Autodesk Inventor part; units mm, degrees
ref_plane "YZ Plane" through (0, 0, 0) normal (1, 0, 0) x (0, 1, 0)
ref_plane "XZ Plane" through (0, 0, 0) normal (0, 1, 0) x (-1, 0, 0)
ref_plane "XY Plane" through (0, 0, 0) normal (0, 0, 1) x (1, 0, 0)
sketch "Sketch1" plane through (0, 0, 0) normal (0, 1, 0) x (-1, 0, 0)
  circle A0 centre (0, 0) radius 36
  circle A1 centre (0, 0) radius 29
  line L0 (0, 0) -> (32.313, 0)
  circle A2 centre (32.313, 0) radius 1.25
  circle A3 centre (16.1565, 27.9839) radius 1.25
  circle A4 centre (-16.1565, 27.9839) radius 1.25
  circle A5 centre (-32.313, 0) radius 1.25
  circle A6 centre (-16.1565, -27.9839) radius 1.25
  circle A7 centre (16.1565, -27.9839) radius 1.25
  dimension "d0" = 72
  dimension "d1" = 58
  dimension "d2" = 32.313
  dimension "d3" = 2.5
  dimension "d6" = 360
extrude "Extrusion1" add sketch "Sketch1" along normal blind 15
sketch "Sketch2" plane through (0, 15, 0) normal (0, 1, 0) x (1, 0, 0)
  circle A0 centre (0, 0) radius 29
  circle A1 centre (0, 0) radius 31.063
  circle A2 centre (-16.1565, 27.9839) radius 1.25
  circle A3 centre (0, 0) radius 36
  point P0 (-15.5315, 26.9013)
extrude "Extrusion2" cut sketch "Sketch2" against normal blind 10 contours A3
sketch "Sketch3" plane through (0, 15, 0) normal (0, 1, 0) x (1, 0, 0)
  circle A0 centre (0, 0) radius 31.063
  circle A1 centre (0, 0) radius 8.5
  dimension "d12" = 17
extrude "Extrusion3" add sketch "Sketch3" along normal blind 3
sketch "Sketch4" plane through (0, 18, 0) normal (0, 1, 0) x (1, 0, 0)
  circle A0 centre (-32.313, 0) radius 1.25
  circle A1 centre (-32.313, 0) radius 3
  circle A2 centre (0, 0) radius 8.5
  circle A3 centre (-16.1565, -27.9839) radius 3
  circle A4 centre (16.1565, -27.9839) radius 3
  circle A5 centre (32.313, 0) radius 3
  circle A6 centre (16.1565, 27.9839) radius 3
  circle A7 centre (-16.1565, 27.9839) radius 3
  dimension "d15" = 6
  dimension "d18" = 360
extrude "Extrusion4" cut sketch "Sketch4" against normal up to surface (13 mm away) contours A0 | A1 | A3 | A4 | A5 | A6 | A7
properties part number "Stage_1_Lid"
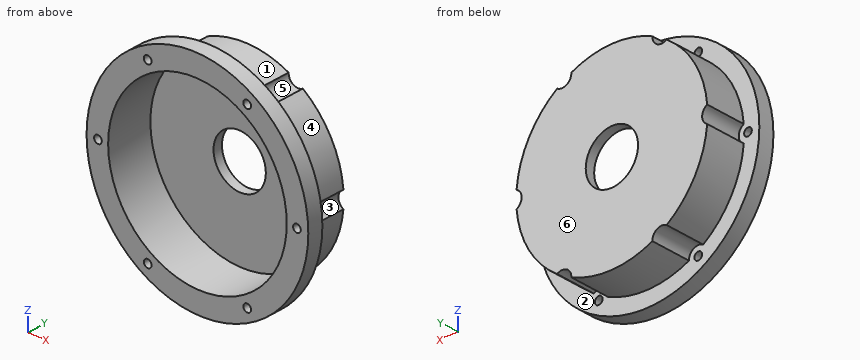
Verification items for the finished model (mm, model axes). Face numbers are marked on the shaded views. A direction names the side the tool comes from. Coordinates: 2 decimals unless noted, no trailing zeros. Write each loop counter-clockwise with the first axis right and the second up, starting at its lowest first coordinate (ties: lowest second). Pieces come first, ordered by that corner, then holes. Notation, with made-up numbers: (76.25, 40.25) -> (91.25, 40.25) arc R7 cw to (91.25, 50.25) -> close; hole circle Ø3 at (67.25, -23.75). An arc over 180 degrees is marked (long way). One line per item, written item: value. Start each with the question number.
Q1. Access from +Z, -Z, +X, -X, +Y, -Y to the whole of each face (thin tool, end or side, straight path). Record for the marked faces 1, 2 and 3.
Q2. Cross-section at A-A on x = 0. Enter the section's corners in (y, z), and give its area (3 significant figures).
Q3. Thickness scan on L1, parallel to X at y = 1, z = 0.5; L2, parallel to Z at x = -12.5, y = 1.5; L3, parallel to Y at x = 19, z = 30.5. Record the ranges inside material, lowest first. Write a range as from..to.
Q4. Cross-section at B-B on y = 16.75. Enter the section's corners in (x, z).
Q5. Go/stop test with flat-tipped pins: P1, Ø2, axis at y = 2.5, z = -11, coming from the -X side; P2, Ø5, axis at y = 9, z = -19.5, coming from the -X side; P3, Ø4, axis at x = -16.16, z = -27.98, coming from the -Y side; P4, Ø1.5, axis at y = 2.5, z = -4.5, coming from the +X side. Record where each tip stops, or that it passes through.
Q6. Mould release check, pull along X, two halves, no side actions. Record for the marked faces 4, 5 and 6: pulls with the +X half, pulls with the -X half, needs draft (parallel to the pull), parting line crosses it, or undercut.
Q7. Cross-section at D-D on y = 1.75. Enter the section's corners in (x, z), and give its area (3 significant figures).
Q8. Cross-section at C-C on z = 0. Enter the section's corners in (x, y), and give its area (3 significant figures).
Checked values:
1. face 1: +Z, +Y
1. face 2: +Y
1. face 3: +X, +Y
2. outline: (0, -36) -> (5, -36) -> (5, -31.06) -> (18, -31.06) -> (18, -8.5) -> (15, -8.5) -> (15, -29) -> (0, -29) -> close; (0, 29) -> (15, 29) -> (15, 8.5) -> (18, 8.5) -> (18, 31.06) -> (5, 31.06) -> (5, 36) -> (0, 36) -> close
2. area: 247 mm²
3. L1: x = -36..-33.46, -31.17..-29, 29..31.17, 33.46..36
3. L2: z = -33.76..-26.17, 26.17..33.76
3. L3: y = 0..5
4. outline: (-30.95, -2.67) arc R31.06 ccw to (-17.79, -25.47) arc R3 cw to (-13.16, -28.14) arc R31.06 ccw to (13.16, -28.14) arc R3 cw to (17.79, -25.47) arc R31.06 ccw to (30.95, -2.67) arc R3 cw to (30.95, 2.67) arc R31.06 ccw to (17.79, 25.47) arc R3 cw to (13.16, 28.14) arc R31.06 ccw to (-13.16, 28.14) arc R3 cw to (-17.79, 25.47) arc R31.06 ccw to (-30.95, 2.67) arc R3 cw to start; hole circle Ø17 at (0, 0)
5. P1: stops at x = -34.58
5. P2: stops at x = -26
5. P3: stops at y = 0
5. P4: stops at x = 35.8
6. face 4: pulls with the +X half
6. face 5: undercut
6. face 6: needs draft
7. outline: circle Ø72 at (0, 0); hole circle Ø2.5 at (-32.31, 0); hole circle Ø58 at (0, 0); hole circle Ø2.5 at (-16.16, -27.98); hole circle Ø2.5 at (-16.16, 27.98); hole circle Ø2.5 at (16.16, -27.98); hole circle Ø2.5 at (16.16, 27.98); hole circle Ø2.5 at (32.31, 0)
7. area: 1,400 mm²
8. outline: (-36, 0) -> (-33.56, 0) -> (-33.56, 5) -> (-36, 5) -> close; (-31.06, 0) -> (-29, 0) -> (-29, 15) -> (-8.5, 15) -> (-8.5, 18) -> (-29.31, 18) -> (-29.31, 5) -> (-31.06, 5) -> close; (8.5, 15) -> (29, 15) -> (29, 0) -> (31.06, 0) -> (31.06, 5) -> (29.31, 5) -> (29.31, 18) -> (8.5, 18) -> close; (33.56, 0) -> (36, 0) -> (36, 5) -> (33.56, 5) -> close
8. area: 176 mm²
